```python
from build123d import *

# Parameters (mm, degrees)
F0_W = 210
F0_H = 210
F3_R = 5


with BuildPart() as f2:
    # F2: sweep along a path in F1
    with BuildLine(Plane.XZ) as f2_path:
        Line((0, 0), (0, 5))
    # F0 (on Top) → F2 (sweep)
    with BuildSketch(Plane.XY):
        Rectangle(F0_W, F0_H)
    sweep(path=f2_path.line)

    # F5: sweep along a path in F4
    with BuildLine(Plane.XZ) as f5_path:
        Line((0, 0), (0, 10))
    # F3 (on Top) → F5 (sweep, cut)
    with BuildSketch(Plane.XY):
        with Locations((-95, -95)):
            Circle(F3_R)
        with Locations((95, 95)):
            Circle(F3_R)
        with Locations((-95, 95)):
            Circle(F3_R)
        with Locations((95, -95)):
            Circle(F3_R)
    sweep(path=f5_path.line, mode=Mode.SUBTRACT)


solid = f2.part
```
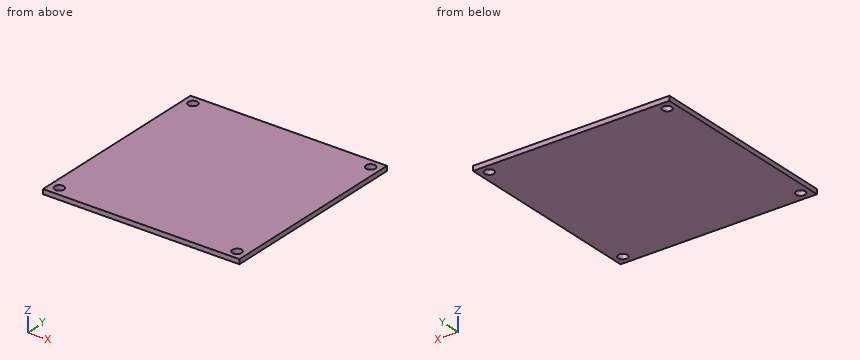
The listing builds one solid part. Answer for the finished solid, in the listing's coordinates (mm). Coordinates: 2 decimals unless noted, no trailing zeros. Write each loop counter-clockwise with the first axis right and the second up, starting at its lowest first coordinate (ties: lowest second). Pieces come first, ordered by that corner, then holes. Notation, with made-up numbers: M -30.75,41 L -16.75,41 A7 cw -16.75,46 Z; hole C 37,-36 d10. An arc over 180 degrees is marked long. Use a Markdown table: item, result. Add a question column.
1. Section A-A (y = -95) is taken. Give the vertices of the cut face in (x, z), plus the area to 3 significant figures.
2. Straight lines are drawn through the part: line 1 along Y through (x, z) = (95, 3.25); line 2 along Y through (x, z) = (-91, 0.7). For each, find the intervals that lie inside material, in ascending order. Write a range as [from, to].
3. Given P1, Ø6, axis at x = -95, y = 95, coming from the +Z side, flat-ended and moving along its own axis, determine where the tip first touches the part or whether it passes through.
Data:
| question | item | result |
|---|---|---|
| 1 | outline | M -105,0 L -100,0 L -100,5 L -105,5 Z; M -90,0 L 90,0 L 90,5 L -90,5 Z; M 100,0 L 105,0 L 105,5 L 100,5 Z |
| 1 | area | 950 mm2 |
| 2 | line 1 | y = [-105, -100], [-90, 90], [100, 105] |
| 2 | line 2 | y = [-105, -98], [-92, 92], [98, 105] |
| 3 | P1 | passes through |
